```python
from build123d import *

# Parameters (mm, degrees)
SKETCH_R     = 6.5
SKETCH_R_2   = 0.936276
PAD_DEPTH    = 1.5
SKETCH001_R  = 0.65
POCKET_DEPTH = 5


with BuildPart() as part:
    # Sketch → Pad (new body)
    with BuildSketch(Plane.XY):
        with Locations((0, 3.563724)):
            Circle(SKETCH_R)
        with Locations((-3.086276, 5.345586)):
            Circle(SKETCH_R_2, mode=Mode.SUBTRACT)
        with Locations((3.086276, 5.345586)):
            Circle(SKETCH_R_2, mode=Mode.SUBTRACT)
        Circle(SKETCH_R_2, mode=Mode.SUBTRACT)
    extrude(amount=PAD_DEPTH)

    # Sketch001 (on Face6 of Pad) → Pocket (cut)
    with BuildSketch(Plane.XY.offset(1.5)):
        with Locations((-3.535534, 3.563724)):
            Circle(SKETCH001_R)
        with Locations((0, 7.099258)):
            Circle(SKETCH001_R)
        with Locations((3.535534, 3.563724)):
            Circle(SKETCH001_R)
        Circle(SKETCH001_R)
    extrude(amount=-POCKET_DEPTH, mode=Mode.SUBTRACT)


with BuildPart() as part_1:
    # Body placement: moved
    add(part.part.moved(Location((20, 0, 0))))


solid = part_1.part
```
Part model, mm, in its own coordinate system. Round coordinates to 2 decimals unless told otherwise and drop trailing zeros. Loops run counter-clockwise (first coordinate to the right, second up) from the corner with the lowest first, then second, coordinate; pieces in that order, holes last.
1. Slice it at A-A (x = 20). Give the cut face in (y, z), and give its area (3 significant figures).
Solutions:
outline: (-2.94, 0) - (-0.94, 0) - (-0.94, 1.5) - (-2.94, 1.5) - close; (0.94, 0) - (6.45, 0) - (6.45, 1.5) - (0.94, 1.5) - close; (7.75, 0) - (10.06, 0) - (10.06, 1.5) - (7.75, 1.5) - close
area: 14.7 mm2
2. Slice it at D-D (y = 9.25). Give the cut face in (x, z).
Solutions:
outline: (16.85, 0) - (23.15, 0) - (23.15, 1.5) - (16.85, 1.5) - close
3. Slice it at C-C (z = 0.6). Give the cut face in (x, y).
Solutions:
outline: circle Ø13 at (20, 3.56); hole circle Ø1.3 at (16.46, 3.56); hole circle Ø1.87 at (16.91, 5.35); hole circle Ø1.87 at (20, 0); hole circle Ø1.3 at (20, 7.1); hole circle Ø1.87 at (23.09, 5.35); hole circle Ø1.3 at (23.54, 3.56)
4. Slice it at B-B (y = 0). Give the cut face in (x, z), and give its area (3 significant figures).
Solutions:
outline: (14.56, 0) - (19.06, 0) - (19.06, 1.5) - (14.56, 1.5) - close; (20.94, 0) - (25.44, 0) - (25.44, 1.5) - (20.94, 1.5) - close
area: 13.5 mm2
5. Drill centre lines: line 1 along Y through (x, z) = (20, 0.35); line 2 along X through (y, z) = (3.5, 1); line 3 along X through (y, z) = (6, 1.4). Where is each one in solid material? Low to high.
Solutions:
line 1: y = -2.94 to -0.94, 0.94 to 6.45, 7.75 to 10.06
line 2: x = 13.5 to 15.82, 17.11 to 22.89, 24.18 to 26.5
line 3: x = 13.97 to 16.24, 17.58 to 22.42, 23.76 to 26.03
